Design review of the part shown in the three views and the two pictorial views. Dimensions are in mm from the part's minimum x, y and z. A direction names the side the tool comes from. Round coordinates to 2 decimals unless told otherwise and drop trailing zeros. Loops run counter-clockwise (first coordinate to the right, second up) from the corner with the lowest first, then second, coordinate; pieces in that order, holes last. Notation, with made-up numbers: M 4,-14.75 L 16,-14.75 A24 ccw 16,19.25 Z; hole C 30,39 d2. An arc over 180 degrees is marked long. Return JSON: item names as keys, results as strings. Group by question number.
Q1. Consider section B-B (y = 3.25). State the section outline as (x, z) points.
Q2. Consider section A-A (z = 3.8). State the section outline as (x, y) points.
Q3. Consider section C-C (x = 3.8). State the section outline as (y, z) points.
Q4. To check wall thickness, follow line 1 along Z through (x, y) = (6, 6.75); line 2 along Z through (x, y) = (2.5, 5.5); line 3 along X through (y, z) = (6, 2.75). State the ranges of each line that lie inside material, in increasing order.
Q5. Draft analysis for pull direction X (two halves, no side actions). For the marked faces 3, 4 and 5, state which applies: pulls with the +X half, pulls with the -X half, needs draft (parallel to the pull), parting line crosses it, or undercut.
Q6. For the marked faces 1 and 2, list the 3-axis set-ups (+Z, -Z, +X, -X, +Y, -Y) from which the entire face can be reached by the end or side of a thin tool; tool diameter is ignored.
Q7. Clearance check with flat-ended pins moving along their axes: pin 1 Ø1.9 at (x, y) = (4, 3) entering from +Z; pin 2 Ø0.6 at (x, y) = (6, 2) entering from -Z; pin 3 Ø1.3 at (x, y) = (6, 5) entering from +Z; pin 4 Ø1.3 at (x, y) = (2, 4.5) entering from -Z. State where each tip first meets the part, or that it passes through.
Q8. Consider section D-D (z = 7.25). State the section outline as (x, y) points, and give its area (3 significant figures).
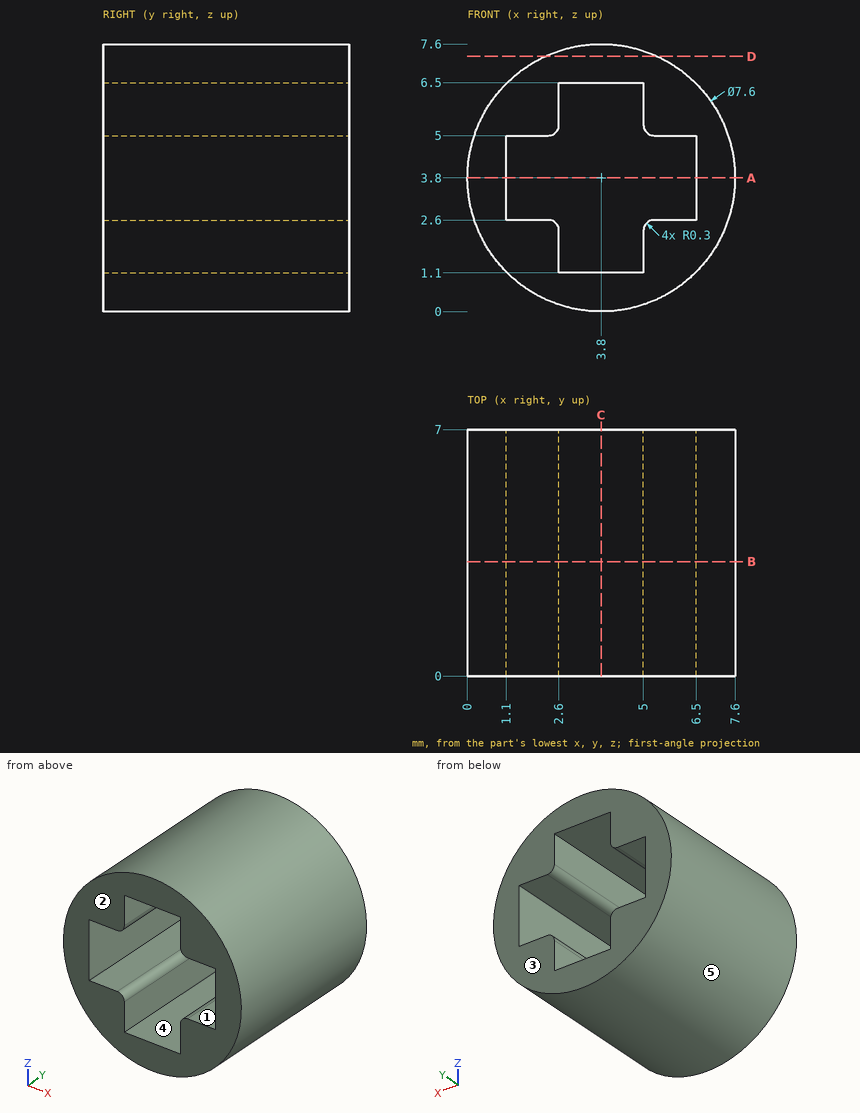
Values:
{
 "1": {"outline": "C 3.8,3.8 d7.6; hole M 1.1,2.6 L 2.3,2.6 A0.3 cw 2.6,2.3 L 2.6,1.1 L 5,1.1 L 5,2.3 A0.3 cw 5.3,2.6 L 6.5,2.6 L 6.5,5 L 5.3,5 A0.3 cw 5,5.3 L 5,6.5 L 2.6,6.5 L 2.6,5.3 A0.3 cw 2.3,5 L 1.1,5 Z"},
 "2": {"outline": "M 0,0 L 1.1,0 L 1.1,7 L 0,7 Z; M 6.5,0 L 7.6,0 L 7.6,7 L 6.5,7 Z"},
 "3": {"outline": "M 0,0 L 7,0 L 7,1.1 L 0,1.1 Z; M 0,6.5 L 7,6.5 L 7,7.6 L 0,7.6 Z"},
 "4": {"line 1": "z = 0.7 to 2.6, 5 to 6.9", "line 2": "z = 0.23 to 2.52, 5.08 to 7.37", "line 3": "x = 0.15 to 1.1, 6.5 to 7.45"},
 "5": {"face 3": "needs draft", "face 4": "undercut", "face 5": "parting line crosses it"},
 "6": {"face 1": "+Y, -Y", "face 2": "+Z, -Z, +X, -X, -Y"},
 "7": {"pin 1": "stops at z = 7.6", "pin 2": "stops at z = 0.51", "pin 3": "stops at z = 7.27", "pin 4": "stops at z = 0.18"},
 "8": {"outline": "M 2.21,0 L 5.39,0 L 5.39,7 L 2.21,7 Z", "area": "22.3 mm2"}
}
